Verification items for this drawing (mm, ordinates from the low corner). A direction names the side the tool comes from. Round coordinates to 2 decimals unless told otherwise and drop trailing zeros. Order: outer loops, then holes, each group sorted by start corner. A loop starts at its lowest first (then second) coordinate and runs counter-clockwise, first axis right, second up.
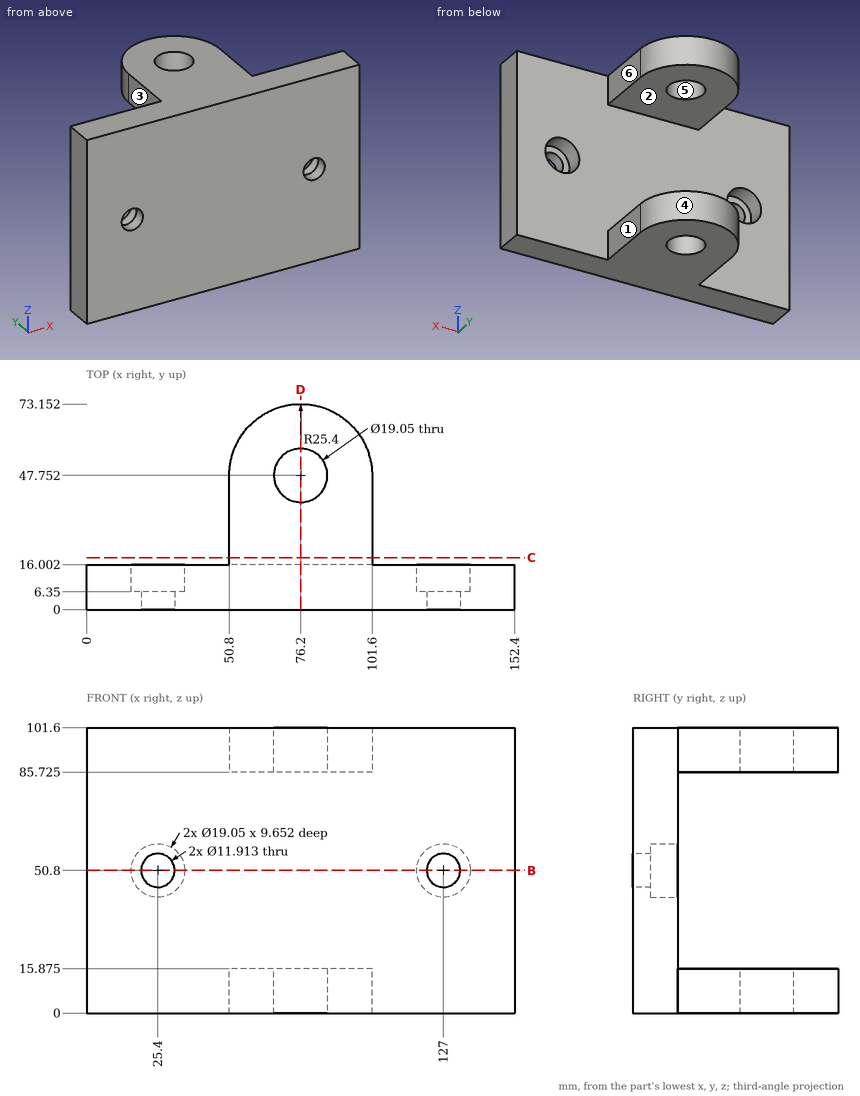
Item 1: Sectioned sample at B-B (z = 50.8). State how many separate pieces and enclosed holes the cut face has, and give its area (3 significant figures).
Answer:
separate pieces: 3
enclosed holes: 0
area: 1,920 mm2
Item 2: Scan lines: line 1 along X through (y, z) = (11, 50); line 2 along X through (y, z) = (1.5, 50.8); line 3 along Z through (x, y) = (84, 35) (1 decimal). Record each from-to range of solid material in increasing order.
Answer:
line 1: x = 0 to 15.91, 34.89 to 117.51, 136.49 to 152.4
line 2: x = 0 to 19.44, 31.36 to 121.04, 132.96 to 152.4
line 3: z = 0 to 15.9, 85.7 to 101.6
Item 3: Sectioned sample at D-D (x = 76.2). Record the cut outline in (y, z) (1 decimal).
Answer:
outline: (0, 0) - (38.2, 0) - (38.2, 15.9) - (16, 15.9) - (16, 85.7) - (38.2, 85.7) - (38.2, 101.6) - (0, 101.6) - close; (57.3, 0) - (73.2, 0) - (73.2, 15.9) - (57.3, 15.9) - close; (57.3, 85.7) - (73.2, 85.7) - (73.2, 101.6) - (57.3, 101.6) - close
Item 4: Release check for a two-part mould opening along Y. For the marked faces 4, 5 and 6 record: released by +Y, released by -Y, zero draft, split by the parting line, or undercut.
Answer:
face 4: released by +Y
face 5: undercut
face 6: zero draft
Item 5: Go/stop test with flat-tipped pins: P1, Ø17.5, axis at y = 38.5, z = 94.5, coming from the -X side; P2, Ø11.5, axis at x = 127, z = 50.8, coming from the +Y side; P3, Ø6, axis at x = 86, z = 44, coming from the +Y side; P4, Ø17.5, axis at y = 30, z = 4, coming from the +X side. Record where each tip stops, or that it passes through.
Answer:
P1: stops at x = 50.8
P2: passes through
P3: stops at y = 16
P4: stops at x = 101.6
Item 6: Sectioned sample at C-C (y = 18.5). Record the cut outline in (x, z) (1 decimal), and give its area (3 significant figures).
Answer:
outline: (50.8, 0) - (101.6, 0) - (101.6, 15.9) - (50.8, 15.9) - close; (50.8, 85.7) - (101.6, 85.7) - (101.6, 101.6) - (50.8, 101.6) - close
area: 1,610 mm2
Item 7: Access from +Z, -Z, +X, -X, +Y, -Y to the whole of each face (thin tool, end or side, straight path). Record for the marked faces 1, 2 and 3.
Answer:
face 1: +Z, -Z, +X, +Y
face 2: +X, -X, +Y
face 3: +Z, -Z, -X, +Y
